Source: CAD feature listing. Evaluate the final solid. Frame: model axes, mm. Face numbers are marked on the shaded views. Coordinates: 2 decimals unless noted, no trailing zeros. Write each loop counter-clockwise with the first axis right and the second up, starting at its lowest first coordinate (ties: lowest second). Pieces come first, ordered by that corner, then holes. Notation, with made-up numbers: (29.5, 88) - (63.5, 88) arc R34 cw to (63.5, 120) - close; hole circle Ø10 at (62.25, 18). An arc over 180 degrees is marked (long way). One line per item, written item: value.
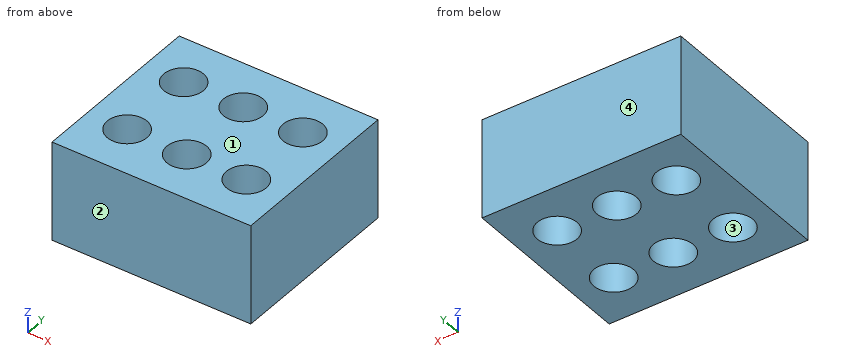
from build123d import *

# Parameters (mm, degrees)
CYLINDER001_R     = 2
CYLINDER001_DEPTH = 10
CYLINDER002_R     = 2
CYLINDER002_DEPTH = 10
CYLINDER_R        = 2
CYLINDER_DEPTH    = 10
BOX_W             = 20
BOX_H             = 10
BOX_DEPTH         = 10
CYLINDER004_R     = 2
CYLINDER004_DEPTH = 10
CYLINDER005_R     = 2
CYLINDER005_DEPTH = 10
CYLINDER003_R     = 2
CYLINDER003_DEPTH = 10
BOX001_W          = 20
BOX001_H          = 10
BOX001_DEPTH      = 10


with BuildPart() as cylinder001:
    # Cylinder001 → Cylinder001 (new body)
    with BuildSketch(Plane(origin=(10, 5, 0), x_dir=(1, 0, 0), z_dir=(0, 0, 1))):
        Circle(CYLINDER001_R)
    extrude(amount=CYLINDER001_DEPTH)


with BuildPart() as cylinder002:
    # Cylinder002 → Cylinder002 (new body)
    with BuildSketch(Plane(origin=(16, 5, 0), x_dir=(1, 0, 0), z_dir=(0, 0, 1))):
        Circle(CYLINDER002_R)
    extrude(amount=CYLINDER002_DEPTH)


with BuildPart() as cylinder:
    # Cylinder → Cylinder (new body)
    with BuildSketch(Plane(origin=(4, 5, 0), x_dir=(1, 0, 0), z_dir=(0, 0, 1))):
        Circle(CYLINDER_R)
    extrude(amount=CYLINDER_DEPTH)


with BuildPart() as cut002:
    # Box → Box (new body)
    with BuildSketch(Plane.XY):
        with Locations((10, 5)):
            Rectangle(BOX_W, BOX_H)
    extrude(amount=BOX_DEPTH)

    # Cut: cut Cylinder
    add(cylinder.part, mode=Mode.SUBTRACT)

    # Cut001: cut Cylinder002
    add(cylinder002.part, mode=Mode.SUBTRACT)

    # Cut002: cut Cylinder001
    add(cylinder001.part, mode=Mode.SUBTRACT)


with BuildPart() as cut002_1:
    # Cut002 placement: moved
    add(cut002.part.moved(Location((0, 9, 0))))


with BuildPart() as cylinder004:
    # Cylinder004 → Cylinder004 (new body)
    with BuildSketch(Plane(origin=(10, 5, 0), x_dir=(1, 0, 0), z_dir=(0, 0, 1))):
        Circle(CYLINDER004_R)
    extrude(amount=CYLINDER004_DEPTH)


with BuildPart() as cylinder005:
    # Cylinder005 → Cylinder005 (new body)
    with BuildSketch(Plane(origin=(16, 5, 0), x_dir=(1, 0, 0), z_dir=(0, 0, 1))):
        Circle(CYLINDER005_R)
    extrude(amount=CYLINDER005_DEPTH)


with BuildPart() as cylinder003:
    # Cylinder003 → Cylinder003 (new body)
    with BuildSketch(Plane(origin=(4, 5, 0), x_dir=(1, 0, 0), z_dir=(0, 0, 1))):
        Circle(CYLINDER003_R)
    extrude(amount=CYLINDER003_DEPTH)


with BuildPart() as fusion:
    # Box001 → Box001 (new body)
    with BuildSketch(Plane.XY):
        with Locations((10, 5)):
            Rectangle(BOX001_W, BOX001_H)
    extrude(amount=BOX001_DEPTH)

    # Cut003: cut Cylinder003
    add(cylinder003.part, mode=Mode.SUBTRACT)

    # Cut004: cut Cylinder005
    add(cylinder005.part, mode=Mode.SUBTRACT)

    # Cut005: cut Cylinder004
    add(cylinder004.part, mode=Mode.SUBTRACT)


with BuildPart() as fusion_1:
    # Cut005 placement: moved
    add(fusion.part.moved(Location((0, 1, 0))))

    # Fusion: union Cut002
    add(cut002_1.part)


solid = fusion_1.part
1) Section query B-B on x = 10. Output: boundary loops of the cut face in (y, z), then the cut area to 3 significant figures.
Values found:
outline: (1, 0) - (4, 0) - (4, 10) - (1, 10) - close; (8, 0) - (12, 0) - (12, 10) - (8, 10) - close; (16, 0) - (19, 0) - (19, 10) - (16, 10) - close
area: 100 mm2
2) Section query D-D on x = 15. Output: boundary loops of the cut face in (y, z).
Values found:
outline: (1, 0) - (4.27, 0) - (4.27, 10) - (1, 10) - close; (7.73, 0) - (12.27, 0) - (12.27, 10) - (7.73, 10) - close; (15.73, 0) - (19, 0) - (19, 10) - (15.73, 10) - close
3) Section query A-A on y = 6. Output: boundary loops of the cut face in (x, z).
Values found:
outline: (0, 0) - (2, 0) - (2, 10) - (0, 10) - close; (6, 0) - (8, 0) - (8, 10) - (6, 10) - close; (12, 0) - (14, 0) - (14, 10) - (12, 10) - close; (18, 0) - (20, 0) - (20, 10) - (18, 10) - close
4) Contact query for a flat-ended pin moving along its axis: P1, Ø1.5, axis at y = 4.5, z = 2.5, coming from the -X side. Output: stop coordinate, or through.
Values found:
P1: x = 0
5) Section query C-C on z = 4. Output: boundary loops of the cut face in (x, y), then the cut area to 3 significant figures.
Values found:
outline: (0, 1) - (20, 1) - (20, 19) - (0, 19) - close; hole circle Ø4 at (4, 6); hole circle Ø4 at (4, 14); hole circle Ø4 at (10, 6); hole circle Ø4 at (10, 14); hole circle Ø4 at (16, 6); hole circle Ø4 at (16, 14)
area: 285 mm2
6) Draft query along Y for the marked faces 1, 2, 3 and 4. Return one class per face: released by +Y, released by -Y, zero draft, split by the parting line, or undercut.
Values found:
face 1: zero draft
face 2: released by -Y
face 3: undercut
face 4: released by +Y
7) Material intervals for line 1 (Y direction, x = 16, z = 6); line 2 (X direction, y = 13.25, z = 9); line 3 (X direction, y = 6.25, z = 8.25), sorted ascending.
Values found:
line 1: 1 to 4, 8 to 12, 16 to 19
line 2: 0 to 2.15, 5.85 to 8.15, 11.85 to 14.15, 17.85 to 20
line 3: 0 to 2.02, 5.98 to 8.02, 11.98 to 14.02, 17.98 to 20
